Verification items for the finished model (mm, model axes). A direction names the side the tool comes from. Give positions to 0.01 mm unless a question says otherwise; leave off trailing zeros. Order: outer loops, then holes, each group sorted by start corner. A loop starts at its lowest first (then second) coordinate and runs counter-clockwise, first axis right, second up. Notation, with made-up numbers: (-16, 36.25) - (20, 36.25) arc R26 cw to (20, 50.25) - close; hole circle Ø2 at (-37.75, -6). An arc over 180 degrees is marked (long way). Answer as a JSON object with one key per item and string values.
```python
from build123d import *

# Parameters (mm, degrees)
F0_R     = 76.0385345631
F1_DEPTH = 59.182
F2_R     = 5.08
F3_R     = 5.08
F4_T     = -2.54


# Not quite as in the source:
# - a shell that OpenCascade refuses in one call is made with other operations: the cavity is built on its own and cut out


with BuildPart() as f1:
    # F0 (on Right) → F1 (new body)
    with BuildSketch(Plane.YZ):
        Circle(F0_R)
    extrude(amount=F1_DEPTH)

    # F2
    f2_edges = [f1.edges().sort_by_distance(p)[0] for p in [
        (59.182, -76.038535, 0),
    ]]
    fillet(f2_edges, radius=F2_R)

    # F3
    f3_edges = [f1.edges().sort_by_distance(p)[0] for p in [
        (0, -76.038535, 0),
    ]]
    fillet(f3_edges, radius=F3_R)

    # F4: a shell. OpenCascade refuses it in one call, so the cavity is built on its own and cut out:
    # the body offset inwards by the wall thickness, plus a prism from it out through each open face.
    f4_core = offset(f1.part, amount=F4_T, mode=Mode.PRIVATE)
    f4_exits = [f4_core.faces().sort_by_distance(p)[0] for p in [
        (56.642, 0, 0),
    ]]
    add(f4_core, mode=Mode.SUBTRACT)
    extrude(f4_exits, amount=-F4_T, mode=Mode.SUBTRACT)


solid = f1.part
```
(1) Section check A-A (z = 0). Record the cut outline in (x, y), then the cut area to 3 significant figures.
Computed values:
{"outline": "(0, -70.96) arc R5.08 ccw to (5.08, -76.04) - (54.1, -76.04) arc R5.08 ccw to (59.18, -70.96) - (56.64, -70.96) arc R2.54 cw to (54.1, -73.5) - (5.08, -73.5) arc R2.54 cw to (2.54, -70.96) - (2.54, 70.96) arc R2.54 cw to (5.08, 73.5) - (54.1, 73.5) arc R2.54 cw to (56.64, 70.96) - (59.18, 70.96) arc R5.08 ccw to (54.1, 76.04) - (5.08, 76.04) arc R5.08 ccw to (0, 70.96) - close", "area": "670 mm²"}
(2) Gauge pin test, flat ends, axial feed: pin 1 Ø4 at (x, z) = (50, -14) entering from +Y; pin 2 Ø2 at (x, z) = (33.5, -36.5) entering from +Y; pin 3 Ø8 at (x, z) = (6.5, -6) entering from -Y. Record the tip position at first contact, or that the pin passes through.
Computed values:
{"pin 1": "stops at y = 75.09", "pin 2": "stops at y = 67.24", "pin 3": "stops at y = -76.01"}
(3) Release check for a two-part mould opening along Z. For faces 3 (the flat face through (2.54, -1, 1)), 4 (the flat face through (0, -1, 1)), 5 (the cylindrical face through (29.248, 72.527, 22.84)) record: pulls with the +Z half, pulls with the -Z half, needs draft (parallel to the pull), parting line crosses it, or undercut.
Computed values:
{"face 3": "undercut", "face 4": "needs draft", "face 5": "parting line crosses it"}
(4) Section check C-C (x = 8.5). Record the cut outline in (y, z), then the cut area to 3 significant figures.
Computed values:
{"outline": "circle Ø152.08 at (0, 0); hole circle Ø147 at (0, 0)", "area": "1,190 mm²"}
(5) Material ranges on line 1 along Z through (x, y) = (30, 0); line 2 along Y through (x, z) = (22, -1); line 3 along X through (y, z) = (48.5, -32.5), recorded low to high. Write a range as [from, to].
Computed values:
{"line 1": "z = [-76.04, -73.5], [73.5, 76.04]", "line 2": "y = [-76.03, -73.49], [73.49, 76.03]", "line 3": "x = [0, 2.54]"}
(6) Access from +Z, -Z, +X, -X, +Y, -Y to the whole of each face (thin tool, end or side, straight path). Record for faces 1 (the cylindrical face through (29.25, -58.33, -44.72)), 2 (the cylindrical face through (57.894, 65.548, -27.178)).
Computed values:
{"face 1": "none", "face 2": "+X"}
